Autodesk Inventor part; units mm, degrees
ref_plane "YZ Plane" through (0, 0, 0) normal (1, 0, 0) x (0, 1, 0)
ref_plane "XZ Plane" through (0, 0, 0) normal (0, 1, 0) x (-1, 0, 0)
ref_plane "XY Plane" through (0, 0, 0) normal (0, 0, 1) x (1, 0, 0)
sketch "Sketch1" plane through (0, 0, 0) normal (0, 1, 0) x (-1, 0, 0)
  line L0 (0, -12.6) -> (0, 12.6)
  line L1 (35.5, -9) -> (0, -9)
  line L2 (0, -9) -> (0, 9)
  line L3 (0, 9) -> (35.5, 9)
  line L4 (35.5, 9) -> (35.5, -9)
  line L5 (0, 0) -> (0, -9)
  line L6 (0, 0) -> (0, -9)
  line L7 (55.6, 0) -> (-85.1, 0)
  line L8 (0, -9) -> (-65, -9)
  line L9 (-65, -9) -> (-65, 3)
  line L10 (-65, 3) -> (0, 3)
  line L11 (0, 3) -> (0, -9)
  point P0 (0, 0)
  dimension "d53" = 18
  dimension "d54" = 35.5
  dimension "d56" = 6
  dimension "d57" = 65
extrude "Extrusion3" add sketch "Sketch1" along normal blind 6
sketch "Sketch4" plane through (0, 6, 0) normal (0, 1, 0) x (1, 0, 0)
  line L0 (-35.5, 9) -> (-35.5, -9)
  line L1 (-35.5, -9) -> (0, -9)
  line L2 (0, -9) -> (0, -3)
  line L3 (0, -3) -> (65, -3)
  line L4 (65, -3) -> (65, 9)
  line L5 (65, 9) -> (-35.5, 9)
  line L6 (0, 12.6) -> (0, -12.6)
  line L7 (-55.6, 0) -> (85.1, 0)
  line L8 (-29.5, 3.5) -> (-6, 3.5)
  line L9 (-6, 3.5) -> (-6, -9)
  line L10 (-6, -9) -> (-29.5, -9)
  line L11 (-29.5, -9) -> (-29.5, 3.5)
  line L12 (-35.5, -9) -> (0, -9)
  line L13 (65, 9) -> (-35.5, 9)
  line L14 (20, 9) -> (65, 0)
  point P0 (0, 0)
  point P1 (0, 9)
  dimension "d58" = 23.5
  dimension "d59" = 12.5
  dimension "d60" = 6
  dimension "d64" = 20
extrude "Extrusion5" cut sketch "Sketch4" against normal up to next contours L11 L8 L9 L7 | L7 L9 L1 L11 | L5 L4 L14
fillet "Fillet10" radius 40 2 edges at (0, 3, 3) (20, 3, -9)
fillet "Fillet11" radius 2 2 edges at (65, 3, 0) (65, 3, 3)
sketch "Sketch5" plane through (0, 6, 0) normal (0, 1, 0) x (1, 0, 0)
  arc A0 (59.802, -3) -> (60.1942, 0.9612) centre (59.802, -1) ccw
  line L0 (60.1942, 0.9612) -> (23.8839, 8.2232)
  arc A1 (23.8839, 8.2232) -> (16.0392, 9) centre (16.0392, -31) ccw
  line L1 (16.0392, 9) -> (-35.5, 9)
  line L2 (-35.5, 9) -> (-35.5, -9)
  line L3 (-35.5, -9) -> (-29.5, -9)
  line L4 (-29.5, -9) -> (-29.5, 3.5)
  line L5 (-29.5, 3.5) -> (-6, 3.5)
  line L6 (-6, 3.5) -> (-6, -9)
  line L7 (-6, -9) -> (0, -9)
  arc A2 (21.0713, -3) -> (0, -9) centre (21.0713, -43) ccw
  line L8 (21.0713, -3) -> (59.802, -3)
  line L9 (0, 19.6325) -> (0, -53.4387)
  line L10 (-55.6, 0) -> (85.1, 0)
  point P0 (0, 0)
  point P1 (-32, -3)
  point P2 (-3.5, -3)
  dimension "d69" = 6
  dimension "d70" = 6
  dimension "d71" = 2.5
  dimension "d72" = 2.5
hole "Hole3" at (-32, 6, 3) at (-3.5, 6, 3) direction (0, -1, 0) diameter 2 depth 2.5
fillet "Fillet12" radius 4 1 edges at (-35.5, 3, -9)
fillet "Fillet13" radius 1 14 edges at (19.9807, 0, -8.8053) (40.4371, 0, 3) (61.7931, 0, 1.1972) (42.0395, 0, -4.5921) (-7.7304, 0, -9) (-34.3284, 0, -7.8284) (-35.5, 0, 2) (-34.3284, 6, -7.8284) (-35.5, 6, 2) (19.9807, 6, -8.8053) (42.0395, 6, -4.5921) (61.7931, 6, 1.1972) (40.4371, 6, 3) (-7.7304, 6, -9)
properties part number "tibia_v3"
Source: CAD feature listing. Evaluate the final solid. Frame: model axes, mm. A direction names the side the tool comes from. Round coordinates to 2 decimals unless told otherwise and drop trailing zeros. Loops run counter-clockwise (first coordinate to the right, second up) from the corner with the lowest first, then second, coordinate; pieces in that order, holes last.
(1) Section query A-A (x = -3.5). Output: boundary loops of the cut face in (y, z).
From the geometry:
outline: (0, -8) arc R1 ccw to (1, -9) - (5, -9) arc R1 ccw to (6, -8) - (6, 2) - (3.5, 2) - (3.5, 4) - (6, 4) - (6, 9) - (0, 9) - close
(2) Access query for faces 4 (the cylindrical face through (-4.49, 4.73, 2.87)), 5 (the flat face through (-6, 3, 3)), 6 (the flat face through (41, 3, 3)), 7 (the cylindrical face through (20.04, 3.03, -8.8)), 8 (the flat face through (-32, 3, 9)). Directions: +Z, -Z, +X, -X, +Y, -Y. A direction counts if a zero-diameter tool reaches every point of the face in a straight line with its end or side. Return the directions, or none.
From the geometry:
face 4: +Y
face 5: +Z, +Y, -Y
face 6: +Z, +X, +Y, -Y
face 7: -Z, +X, +Y, -Y
face 8: +Z, +X, -X, +Y, -Y
(3) Material intervals for probe 1 along Z at (x, y) = (-3.5, 4.6); probe 2 along X at (y, z) = (4.25, 2.25); probe 3 along Z at (x, y) = (35, 3.5), sorted ascending.
From the geometry:
probe 1: z = -9 to 2, 4 to 9
probe 2: x = -35.5 to -32.66, -31.34 to -29.5, -6 to -4.16, -2.84 to 61.36
probe 3: z = -6 to 3
(4) Section query B-B (x = -27). Output: boundary loops of the cut face in (y, z).
From the geometry:
outline: (0, -8) arc R1 ccw to (1, -9) - (5, -9) arc R1 ccw to (6, -8) - (6, -3.5) - (0, -3.5) - close
(5) Pull-direction query (Z, two-part tool) for faces 1 (the cylindrical face through (-33, 5, 3)), 2 (the flat face through (-8, 3, -9)), 3 (the cylindrical face through (9.97, 2.97, 4.57)); classes: +Z half, -Z half, draft (parallel to the pull), parting line (faces both ways), or undercut.
From the geometry:
face 1: undercut
face 2: -Z half
face 3: +Z half
(6) Contact query for flat-ended pins moving along their axis: pin 1 Ø1.2 at (x, y) = (44.5, 2) entering from +Z; pin 2 Ø4 at (x, z) = (51, -5) entering from -Y; pin 3 Ø3 at (x, y) = (-21, 3) entering from +Z; pin 4 Ø0.6 at (x, z) = (-32, 3) entering from +Y. Output: stop coordinate, or through.
From the geometry:
pin 1: stops at z = 3
pin 2: passes through
pin 3: stops at z = -3.5
pin 4: stops at y = 3.5
